```python
from build123d import *

# Parameters (mm, degrees)
F1_DEPTH = 12.7


with BuildPart() as f1:
    # F0 (on Front) → F1 (new body)
    with BuildSketch(Plane.XZ):
        with BuildLine():
            ThreePointArc((126.608238, -33.298336), (63.743612, -11.900326), (-2.618616, -9.473213))
            ThreePointArc((-2.618616, -9.473213), (-18.720598, -18.239824), (-22.427845, -36.194868))
            ThreePointArc((-22.427845, -36.194868), (-19.702387, -40.069858), (-15.053131, -40.979846))
            ThreePointArc((-15.053131, -40.979846), (60.218564, -39.206701), (131.983539, -61.983018))
            ThreePointArc((131.983539, -61.983018), (139.438808, -60.744668), (140.429628, -53.252484))
            ThreePointArc((140.429628, -53.252484), (134.91852, -44.025519), (128.818874, -35.176593))
            ThreePointArc((128.818874, -35.176593), (127.822247, -34.10954), (126.608238, -33.298336))
        make_face()
    extrude(amount=F1_DEPTH)


solid = f1.part
```
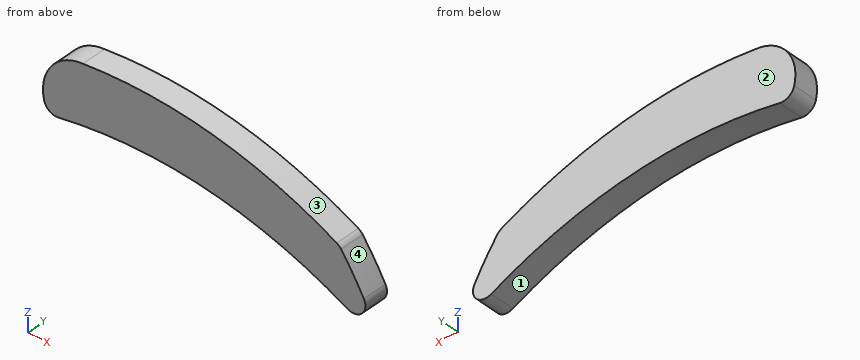
Could you check a few things on this model? Use its own coordinates, in mm. Face numbers are marked on the shaded views. Round coordinates to 2 decimals unless told otherwise and drop trailing zeros. Loops run counter-clockwise (first coordinate to the right, second up) from the corner with the lowest first, then second, coordinate; pieces in that order, holes last. Notation, with made-up numbers: M -30,-24.5 L 7,-24.5 A11 ccw 7,-13.5 Z; hole C 1.25,30 d8. An arc over 180 degrees is marked long. Put each result on its own line as item: value.
Q1. For pin 1 (5 mm diameter, centred on y = -4, z = -39.5, fed in from +X); pin 2 (2 mm diameter, centred on x = 101.5, y = -3, fed in from +Z); pin 3 (2 mm diameter, centred on y = -9.5, z = -47.5, fed in from +X), each with a flat end and sliding along its axis, tell me the tip position at first contact or that it passes through.
Check result:
pin 1: x = 133.6
pin 2: z = -21.9
pin 3: x = 137.69
Q2. Imagine slicing it at A-A (y = -11). Write out the boundary of the cut face in (x, z), then the cut area to 3 significant figures.
Check result:
outline: M -22.43,-36.19 A6.35 ccw -15.05,-40.98 A228.6 cw 131.98,-61.98 A6.35 ccw 140.43,-53.25 A165.13 ccw 128.82,-35.18 A6.35 ccw 126.61,-33.3 A228.6 ccw -2.62,-9.47 A21.79 ccw Z
area: 4,380 mm2
Q3. I need wall thicknesses on probe 1 along Z at (x, y) = (25.5, -2.25); probe 2 along Z at (x, y) = (7.5, -5.75); probe 3 along X at (y, z) = (-1.75, -58). Which ranges of each line are inside material? Lowest first, please.
Check result:
probe 1: -36.92 to -8.13
probe 2: -37.82 to -8.59
probe 3: 123.8 to 141
Q4. Imagine slicing it at B-B (x = 118.5). Write out the boundary of the cut face in (y, z), then the cut area to 3 significant figures.
Check result:
outline: M -12.7,-55.63 L 0,-55.63 L 0,-29.34 L -12.7,-29.34 Z
area: 334 mm2
Q5. Imagine slicing it at C-C (z = -17.5). Write out the boundary of the cut face in (x, y), then the cut area to 3 significant figures.
Check result:
outline: M -18.15,-12.7 L 87.14,-12.7 L 87.14,0 L -18.15,0 Z
area: 1,340 mm2
Q6. Thinking about a two-plate mould opening in X: for the marked faces 1, 2, 3 and 4, which applies, released by +X, released by -X, zero draft, split by the parting line, or undercut?
Check result:
face 1: undercut
face 2: zero draft
face 3: split by the parting line
face 4: released by +X
